Can you work these out from the model? Positions are in its coordinate system, mm. Face numbers are marked on the shaded views. A direction names the side the tool comes from. Coordinates: 2 decimals unless noted, no trailing zeros. Loops run counter-clockwise (first coordinate to the right, second up) from the corner with the lowest first, then second, coordinate; pieces in that order, holes last.
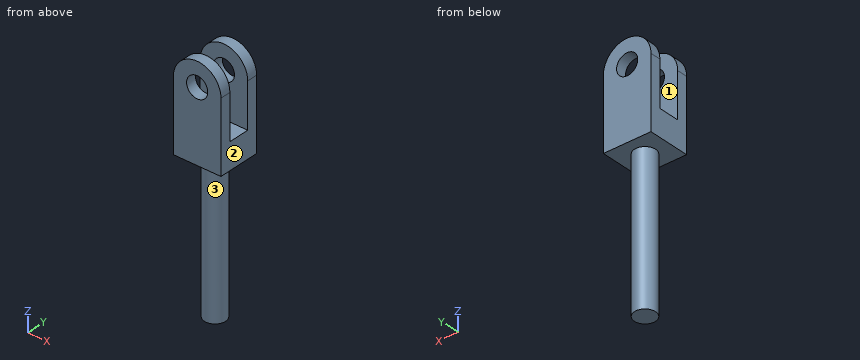
```python
from build123d import *

# Parameters (mm, degrees)
SKETCH1_R          = 12.7
EXTRUDE1_DEPTH     = 177.8
EXTRUDE2_DEPTH     = 28.575
SKETCH3_R          = 12.7
CUT_EXTRUDE1_DEPTH = 298.858323075


with BuildPart() as part:
    # Sketch1 → Extrude1 (new body)
    with BuildSketch(Plane.XY):
        Circle(SKETCH1_R)
    extrude(amount=EXTRUDE1_DEPTH)

    # Sketch2 → Extrude2 (add, symmetric)
    with BuildSketch(Plane(origin=(0, 0, 0), x_dir=(0, 0, -1), z_dir=(1, 0, 0))):
        Polygon((-177.8, -25.4), (-177.8, 25.4), (-292.1, 25.4), (-292.1, 12.7), (-209.55, 12.7), (-209.55, -12.7), (-292.1, -12.7), (-292.1, -25.4), align=None)
    extrude(amount=EXTRUDE2_DEPTH, both=True)

    # Sketch3 → Cut-Extrude1 (cut, through all)
    with BuildSketch(Plane(origin=(0, 25.4, 0), x_dir=(-1, 0, 0), z_dir=(0, 1, 0))):
        with Locations(Location((0, 263.525, 0), (0, 0, 90))):
            Circle(SKETCH3_R)
        with BuildLine():
            Line((28.575, 263.525), (28.575, 314.325))
            Line((28.575, 314.325), (-28.575, 314.325))
            Line((-28.575, 314.325), (-28.575, 263.525))
            ThreePointArc((-28.575, 263.525), (0, 292.1), (28.575, 263.525))
        make_face()
    extrude(amount=-CUT_EXTRUDE1_DEPTH, mode=Mode.SUBTRACT)


solid = part.part
```
Item 1: Suppose I cut it at A-A, the plane x = 0. Please give me the cut outline in (y, z) (3 decimals).
Results are:
outline: (-25.4, 177.8) - (-12.7, 177.8) - (-12.7, 0) - (12.7, 0) - (12.7, 177.8) - (25.4, 177.8) - (25.4, 250.825) - (12.7, 250.825) - (12.7, 209.55) - (-12.7, 209.55) - (-12.7, 250.825) - (-25.4, 250.825) - close; (-25.4, 276.225) - (-12.7, 276.225) - (-12.7, 292.1) - (-25.4, 292.1) - close; (12.7, 276.225) - (25.4, 276.225) - (25.4, 292.1) - (12.7, 292.1) - close
Item 2: Suppose I cut it at D-D, the plane y = 18. Please give me the cut outline in (x, z) (3 decimals), plus the area to 3 significant figures.
Results are:
outline: (-28.575, 177.8) - (28.575, 177.8) - (28.575, 263.525) arc R28.575 ccw to (-28.575, 263.525) - close; hole circle Ø25.4 at (0, 263.525)
area: 5,680 mm2
Item 3: I need wall thicknesses on line 1 along Y through (x, z) = (14.5, 261.5); line 2 along Z through (x, y) = (1, -23); line 3 along Z through (x, y) = (-3, -5). Which ranges of each line are inside material? Lowest first, please.
Results are:
line 1: y = -25.4 to -12.7, 12.7 to 25.4
line 2: z = 177.8 to 250.86, 276.19 to 292.08
line 3: z = 0 to 209.55
Item 4: Suppose I cut it at C-C, the plane y = 0. Please give me the cut outline in (x, z) (3 decimals), plus the area to 3 significant figures.
Results are:
outline: (-28.575, 177.8) - (-12.7, 177.8) - (-12.7, 0) - (12.7, 0) - (12.7, 177.8) - (28.575, 177.8) - (28.575, 209.55) - (-28.575, 209.55) - close
area: 6,330 mm2
Item 5: Suppose I cut it at B-B, the plane z = 260.5. Please give me the cut outline in (x, y) (3 decimals), plus the area to 3 significant figures.
Results are:
outline: (-28.575, -25.4) - (-12.334, -25.4) - (-12.334, -12.7) - (-28.575, -12.7) - close; (-28.575, 12.7) - (-12.334, 12.7) - (-12.334, 25.4) - (-28.575, 25.4) - close; (12.334, -25.4) - (28.575, -25.4) - (28.575, -12.7) - (12.334, -12.7) - close; (12.334, 12.7) - (28.575, 12.7) - (28.575, 25.4) - (12.334, 25.4) - close
area: 825 mm2
Item 6: On a 3-axis mill with a long thin cutter (end or side, diameter ignored), from which of +Z, -Z, +X, -X, +Y, -Y can I reach the whole of each face in a straight line? I mean the marked faces 1, 2 and 3. Say none if no direction works.
Results are:
face 1: +Z, +X, -X
face 2: +Z, -Z, +X, +Y, -Y
face 3: -Z
Item 7: I'm going to push flat-ended pins straight in: P1, Ø6, axis at x = 4.5, y = -4, coming from the -Z side; P2, Ø23, axis at x = 0, z = 263.525, coming from the -Y side; P3, Ø2, axis at x = 7.5, y = -3, coming from the +Z side; P4, Ø10, axis at x = -18, y = 14.5, coming from the +Z side. Where does each tip first touch, or does it pass through?
Results are:
P1: stops at z = 0
P2: passes through
P3: stops at z = 209.55
P4: stops at z = 288.97
